from build123d import *

# Parameters (mm, degrees)
SKETCH_1_W          = 49.8
SKETCH_1_H          = 190
EXTRUDE_1_DEPTH     = 5
SKETCH_3_W          = 30.4
SKETCH_3_H          = 6.3
CUT_EXTRUDE_1_DEPTH = 50


with BuildPart() as part:
    # 草图1 → 凸台-拉伸1 (new, symmetric)
    with BuildSketch(Plane.XY):
        Rectangle(SKETCH_1_W, SKETCH_1_H)
    extrude(amount=EXTRUDE_1_DEPTH, both=True)

    # 草图3 → 切除-拉伸1 (cut)
    with BuildSketch(Plane.XZ.offset(95)):
        Rectangle(SKETCH_3_W, SKETCH_3_H)
    extrude(amount=-CUT_EXTRUDE_1_DEPTH, mode=Mode.SUBTRACT)


solid = part.part
Geometry check sheet. Reference: the model listing, model coordinates, mm. A direction names the side the tool comes from. Give positions to 0.01 mm unless a question says otherwise; leave off trailing zeros. Order: outer loops, then holes, each group sorted by start corner. A loop starts at its lowest first (then second) coordinate and runs counter-clockwise, first axis right, second up. Notation, with made-up numbers: (-22, 10) - (-8, 10) arc R12 cw to (-8, 27) - close; hole circle Ø11 at (59, 45). An arc over 180 degrees is marked (long way). Use one line per item in the form item = value.
1) Access from +Z, -Z, +X, -X, +Y, -Y to the whole of each face (thin tool, end or side, straight path). Record for faces 1 (the face through (-15.2, -70, 0)), 2 (the face through (0, 95, 0)).
Working result:
face_1 = -Y
face_2 = +Z, -Z, +X, -X, +Y
2) Draft check along X on faces 3 (the face through (0, 1, -5)), 4 (the face through (24.9, -1, 0)), 5 (the face through (15.2, -70, 0)), 6 (the face through (0, -70, -3.15)). Enter one of: released by +X, released by -X, zero draft, split by the parting line, or undercut.
Working result:
face_3 = zero draft
face_4 = released by +X
face_5 = undercut
face_6 = undercut
3) Depth check by flat-ended pin: pin 1 Ø1.9 at (x, z) = (-2.5, -1) entering from -Y. Enter the tip coordinate at first touch or a pass-through.
Working result:
pin_1 = -45
4) Sectioned sample at A-A (z = 0). Record the boundary of the cut face in (x, y).
Working result:
outline = (-24.9, -95) - (-15.2, -95) - (-15.2, -45) - (15.2, -45) - (15.2, -95) - (24.9, -95) - (24.9, 95) - (-24.9, 95) - close
5) Material ranges on probe 1 along Z at (x, y) = (9, -70); probe 2 along X at (y, z) = (-64.5, -0.75); probe 3 along Y at (x, z) = (-3.5, 0.5), recorded low to high. Write a range as from..to.
Working result:
probe_1 = -5..-3.15, 3.15..5
probe_2 = -24.9..-15.2, 15.2..24.9
probe_3 = -45..95
6) Sectioned sample at B-B (x = -3). Record the boundary of the cut face in (y, z), and give its area (4 significant figures).
Working result:
outline = (-95, -5) - (95, -5) - (95, 5) - (-95, 5) - (-95, 3.15) - (-45, 3.15) - (-45, -3.15) - (-95, -3.15) - close
area = 1,585 mm^2
